Drawing for the job (mm, zero at the part's lowest x, y, z). A direction names the side the tool comes from. Coordinates: 2 decimals unless noted, no trailing zeros. Write each loop counter-clockwise with the first axis right and the second up, starting at its lowest first coordinate (ties: lowest second). Pieces come first, ordered by that corner, then holes. Notation, with made-up numbers: M 51,35 L 77,35 A22 ccw 77,51 Z; hole C 63.5,35.25 d3. An arc over 180 degrees is marked long. Use a Markdown table: item, result. Add a question column.
Q1. Pin check, flat tips, straight feed: pin 1 Ø1.8 at (y, z) = (9, 9) entering from -X; pin 2 Ø1 at (x, z) = (4, 14) entering from -Y; pin 3 Ø2 at (x, y) = (5.5, 11.5) entering from +Z; pin 4 Ø3 at (x, y) = (6, 12.5) entering from +Z. Stop position of each tip, or through.
Q2. Wall check: L1, parallel to Y at x = 8, z = 9; L2, parallel to X at y = 3, z = 5.25; L3, parallel to Z at x = 5, y = 9.5. Give the ranges that are in metal, low to high. Write a range as from..to.
Q3. Slice it at D-D on z = 15.5. Write the cut outline in (x, y), then the cut area to 3 significant figures.
Q4. Slice it at C-C on x = 12.25. Write the cut outline in (y, z).
Q5. Tool access for the marked faces 1 and 2: list every direction of +Z, -Z, +X, -X, +Y, -Y with a clear straight run to the whole face (end or side of a thin tool).
Q6. Slice it at A-A on y = 9. Write the cut outline in (x, z), then the cut area to 3 significant figures.
Q7. Mould opens along Y. For the marked faces 3, 4 and 5 say: released by +Y, released by -Y, zero draft, split by the parting line, or undercut.
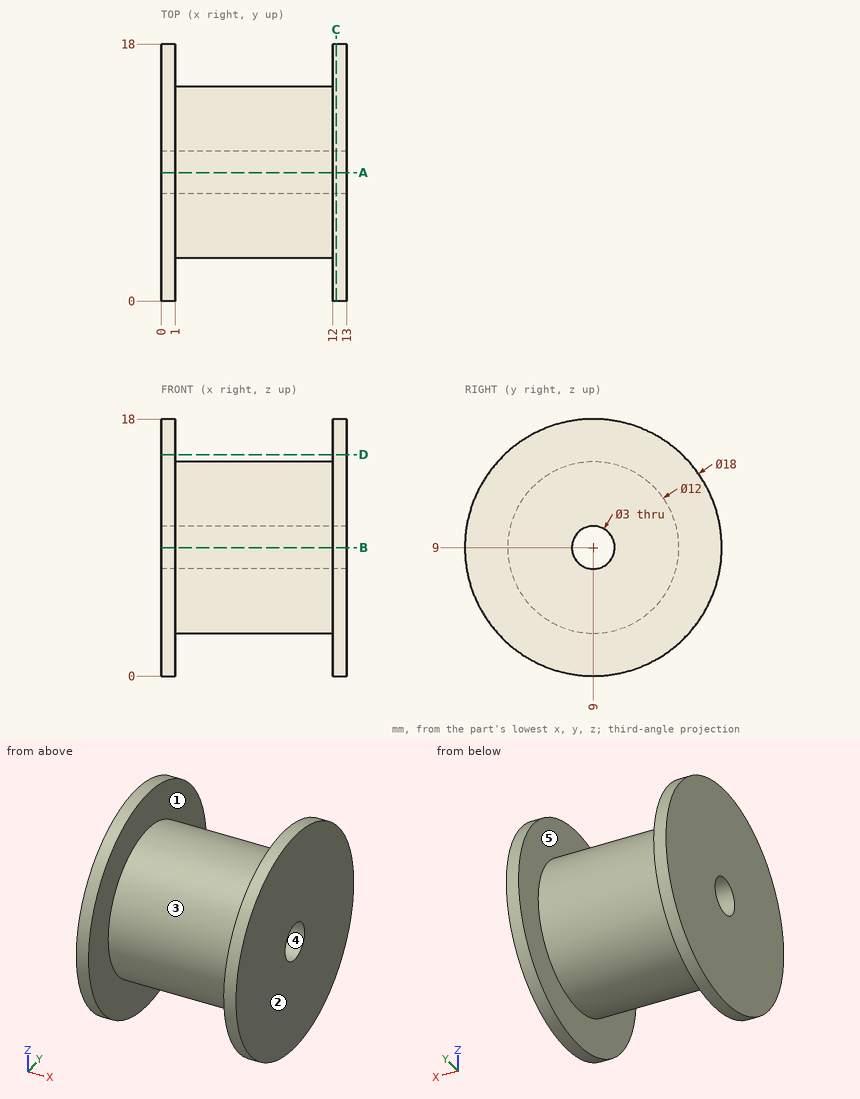
Recorded:
| question | item | result |
|---|---|---|
| 1 | pin 1 | through |
| 1 | pin 2 | y = 5.03 |
| 1 | pin 3 | z = 14.81 |
| 1 | pin 4 | z = 14.66 |
| 2 | L1 | 3..7.5, 10.5..15 |
| 2 | L2 | 0..1, 12..13 |
| 2 | L3 | 3.02..7.59, 10.41..14.98 |
| 3 | outline | M 0,2.78 L 1,2.78 L 1,15.22 L 0,15.22 Z; M 12,2.78 L 13,2.78 L 13,15.22 L 12,15.22 Z |
| 3 | area | 24.9 mm² |
| 4 | outline | C 9,9 d18; hole C 9,9 d3 |
| 5 | face 1 | none |
| 5 | face 2 | +Z, -Z, +X, +Y, -Y |
| 6 | outline | M 0,0 L 1,0 L 1,3 L 12,3 L 12,0 L 13,0 L 13,7.5 L 0,7.5 Z; M 0,10.5 L 13,10.5 L 13,18 L 12,18 L 12,15 L 1,15 L 1,18 L 0,18 Z |
| 6 | area | 129 mm² |
| 7 | face 3 | split by the parting line |
| 7 | face 4 | undercut |
| 7 | face 5 | zero draft |
